Study the drawing (mm; zero at the part's minimum x, y, z) and answer. Round coordinates to 2 decimals unless told otherwise and drop trailing zeros. Order: outer loops, then holes, each group sorted by start corner. A loop starts at its lowest first (then second) coordinate and runs counter-clockwise, first axis right, second up. Notation, with made-up numbers: (-17, 81.5) - (28, 81.5) arc R20 cw to (28, 86.5) - close; hole circle Ø3 at (-7, -8.5). An arc over 180 degrees is marked (long way). Put each result on its own line as item: value. Start each with the question number.
Q1. Section A-A on z = 1.1 is taken. Give the vertices of the cut face in (x, y) (3 decimals), then the cut area to 3 significant figures.
Q2. Section B-B on x = 8.25 is taken. Give the vertices of the cut face in (y, z).
Q3. This flat-tipped pin is pushed along its axis until it touches: pin 1 Ø0.6 at (y, z) = (4, 1) entering from +X. Where does it stop, or does it pass through?
Q4. Find the intervals of material crossed by line 1 along X through (y, z) = (7.25, 1); line 2 along Y through (x, z) = (11.25, 0.55); line 3 along Y through (x, z) = (5.5, 0.25), in increasing order. Write a range as from..to.
Q5. Section C-C on y = 2.75 is taken. Give the vertices of the cut face in (x, z), then the cut area to 3 significant figures.
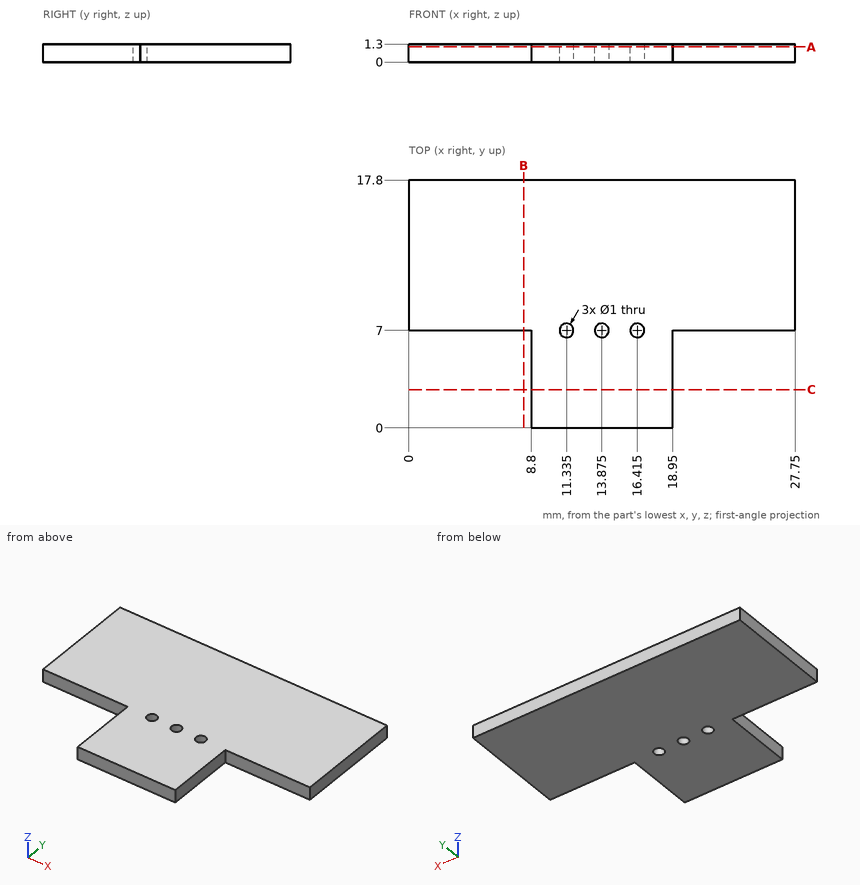
Findings:
1. outline: (0, 7) - (8.8, 7) - (8.8, 0) - (18.95, 0) - (18.95, 7) - (27.75, 7) - (27.75, 17.8) - (0, 17.8) - close; hole circle Ø1 at (11.335, 7); hole circle Ø1 at (13.875, 7); hole circle Ø1 at (16.415, 7)
1. area: 368 mm2
2. outline: (7, 0) - (17.8, 0) - (17.8, 1.3) - (7, 1.3) - close
3. pin 1: x = 18.95
4. line 1: 0..10.9, 11.77..13.44, 14.31..15.98, 16.85..27.75
4. line 2: 0..6.51, 7.49..17.8
4. line 3: 7..17.8
5. outline: (8.8, 0) - (18.95, 0) - (18.95, 1.3) - (8.8, 1.3) - close
5. area: 13.2 mm2
